```python
from build123d import *

# Parameters (mm, degrees)
CYLINDER007_R          = 4
CYLINDER007_DEPTH      = 5
CYLINDER007_ROLL_ANGLE = -90
CYLINDER008_R          = 4
CYLINDER008_DEPTH      = 5
CYLINDER008_ROLL_ANGLE = -90
CHAMFER001_SIZE        = 0.5
BOX014_W               = 36
BOX014_H               = 12
BOX014_DEPTH           = 31
SKETCH013_R            = 2.4
PAD011_DEPTH           = 22
FILLET017_R            = 3
FILLET018_R            = 5
FILLET019_R            = 1


with BuildPart() as cone:
    # Cone → Cone (revolve)
    with BuildSketch(Plane(origin=(53.5, 11, -1), x_dir=(1, 0, 0), z_dir=(0, -1, 0))):
        Polygon((0, 0), (2.2, 0), (4, 15), (0, 15), align=None)
    revolve(axis=Axis((53.5, 11, -1), (0, 0, 1)))


with BuildPart() as cylinder007:
    # Cylinder007 → Cylinder007 (new body)
    with BuildSketch(Plane.XY):
        Circle(CYLINDER007_R)
    extrude(amount=CYLINDER007_DEPTH)


with BuildPart() as cylinder007_1:
    # Cylinder007 roll: moved
    add(cylinder007.part.rotate(Axis((0, 0, 0), (1, 0, 0)), CYLINDER007_ROLL_ANGLE))


with BuildPart() as cylinder007_2:
    # Cylinder007 placement: moved
    add(cylinder007_1.part.moved(Location((22, 15.6, 9))))


with BuildPart() as chamfer001:
    # Cylinder008 → Cylinder008 (new body)
    with BuildSketch(Plane.XY):
        Circle(CYLINDER008_R)
    extrude(amount=CYLINDER008_DEPTH)


with BuildPart() as chamfer001_1:
    # Cylinder008 roll: moved
    add(chamfer001.part.rotate(Axis((0, 0, 0), (1, 0, 0)), CYLINDER008_ROLL_ANGLE))


with BuildPart() as chamfer001_2:
    # Cylinder008 placement: moved
    add(chamfer001_1.part.moved(Location((22, 1.4, 9))))

    # Fusion008: union Cylinder007
    add(cylinder007_2.part)

    # Chamfer001
    chamfer001_edges = [chamfer001_2.edges().sort_by_distance(p)[0] for p in [
        (18, 15.6, 9),
        (18, 6.4, 9),
    ]]
    chamfer(chamfer001_edges, length=CHAMFER001_SIZE)


with BuildPart() as cut022:
    # Box014 → Box014 (new body)
    with BuildSketch(Plane(origin=(-1, 5, -2), x_dir=(1, 0, 0), z_dir=(0, 0, 1))):
        with Locations((18, 6)):
            Rectangle(BOX014_W, BOX014_H)
    extrude(amount=BOX014_DEPTH)

    # Cut022: cut Chamfer001
    add(chamfer001_2.part, mode=Mode.SUBTRACT)


with BuildPart() as cut024:
    # Sketch013 → Pad011 (new body)
    with BuildSketch(Plane.XZ):
        with BuildLine():
            ThreePointArc((10.239335, 25.205378), (1.177797, 22.886123), (2.51191, 13.628125))
            Line((18.823529, 0), (2.51191, 13.628125))
            Line((62, 0), (18.823529, 0))
            Line((62, 10.5), (62, 0))
            Line((25, 17.5), (62, 10.5))
            Line((10.239335, 25.205378), (25, 17.5))
        make_face()
        with Locations((7, 19)):
            Circle(SKETCH013_R, mode=Mode.SUBTRACT)
        with Locations((22, 9)):
            Circle(SKETCH013_R, mode=Mode.SUBTRACT)
    extrude(amount=-PAD011_DEPTH)

    # Cut023: cut Cut022
    add(cut022.part, mode=Mode.SUBTRACT)

    # Fillet017
    fillet017_edges = [cut024.edges().sort_by_distance(p)[0] for p in [
        (18.823529, 2.5, 0),
        (18.823529, 19.5, 0),
        (62, 11, 0),
        (62, 11, 10.5),
    ]]
    fillet(fillet017_edges, radius=FILLET017_R)

    # Fillet018
    fillet018_edges = [cut024.edges().sort_by_distance(p)[0] for p in [
        (35, 11, 0),
        (35, 11, 15.608108),
    ]]
    fillet(fillet018_edges, radius=FILLET018_R)

    # Fillet019
    fillet019_edges = [cut024.edges().sort_by_distance(p)[0] for p in [
        (1.177797, 0, 22.886123),
        (1.177797, 22, 22.886123),
    ]]
    fillet(fillet019_edges, radius=FILLET019_R)

    # Cut024: cut Cone
    add(cone.part, mode=Mode.SUBTRACT)


solid = cut024.part
```
Geometry: final body of the model. Coordinates: model frame, mm. A direction names the side the tool comes from. Coordinates: 2 decimals unless noted, no trailing zeros. Loops run counter-clockwise (first coordinate to the right, second up) from the corner with the lowest first, then second, coordinate; pieces in that order, holes last. Notation, with made-up numbers: (6.5, 21.5) -> (29.5, 21.5) arc R14 ccw to (29.5, 39.5) -> close; hole circle Ø1 at (4.25, 85.25). An arc over 180 degrees is marked (long way). Use a Markdown table: item, result. Add a question column.
(1) Access query for faces 4 (the flat face through (35, 11, 7)), 5 (the cylindrical face through (18.8, 5.4, 11.4)), 6 (the cylindrical face through (10.54, 0.3, 7.29)). Directions: +Z, -Z, +X, -X, +Y, -Y. A direction counts if a zero-diameter tool reaches every point of the face in a straight line with its end or side. Return the directions, or none.
(2) Section query A-A, the plane y = 20.25. Return loops of the section in (x, z).
(3) Pin query (flat end, axial travel): pin 1 Ø2.5 at (y, z) = (9, 8.5) entering from -X; pin 2 Ø1 at (y, z) = (17.5, 14) entering from -X; pin 3 Ø1 at (y, z) = (4.5, 8.5) entering from -X. Return the tip coordinate at first contact, or that it passes through.
(4) Mould query, pull axis Y, two halves, no side actions, for faces 1 (the cylindrical face through (61.1, 11.14, 0.86)), 2 (the flat face through (20, 5, 13)), 3 (the cylindrical face through (41.91, 0.3, 14.01)). Classes: pulls with the +Y half, pulls with the -Y half, needs draft (parallel to the pull), parting line crosses it, or undercut.
(5) Section query B-B, the plane z = 9. State how many separate pieces and enclosed holes the cut face has, plus the area to 3 significant figures.
(6) Line query: line 1 along Y through (x, z) = (28.5, 5.75); line 2 along Z through (x, y) = (22, 2.75); line 3 along Y through (x, z) = (53, 12). Output: solid intervals per line, ascending.
Answer:
| question | item | result |
|---|---|---|
| 1 | face 4 | +Z, -Z |
| 1 | face 5 | none |
| 1 | face 6 | -Z, -X, -Y |
| 2 | outline | (2.51, 13.63) -> (17.99, 0.7) arc R3 ccw to (19.91, 0) -> (59, 0) arc R3 ccw to (62, 3) -> (62, 8.01) arc R3 ccw to (59.56, 10.96) -> (25, 17.5) -> (10.24, 25.21) arc R7 ccw to start; hole circle Ø4.8 at (7, 19); hole circle Ø4.8 at (22, 9) |
| 3 | pin 1 | stops at x = 35 |
| 3 | pin 2 | stops at x = 1.64 |
| 3 | pin 3 | stops at x = 8.05 |
| 4 | face 1 | needs draft |
| 4 | face 2 | undercut |
| 4 | face 3 | pulls with the -Y half |
| 5 | separate pieces | 3 |
| 5 | enclosed holes | 1 |
| 5 | area | 783 mm^2 |
| 6 | line 1 | y = 0 to 5, 17 to 22 |
| 6 | line 2 | z = 0 to 6.6, 11.4 to 19.07 |
| 6 | line 3 | y = 0.4 to 7.27, 14.73 to 21.6 |
